The model under review builds one solid part; all positions refer to its coordinate system, in mm. A direction names the side the tool comes from. Give positions to 0.01 mm unless a question says otherwise; leave off trailing zeros. Loops run counter-clockwise (first coordinate to the right, second up) from the corner with the lowest first, then second, coordinate; pieces in that order, holes last. Notation, with made-up numbers: M 1,-11 L 46,-11 A20 ccw 46,22 Z; hole C 9.5,-0.75 d2. An arc over 180 degrees is marked long. Return JSON: item names as keys, results as strings.
```python
from build123d import *

# Parameters (mm, degrees)
F1_DEPTH      = 1200
F2_W          = 30
F2_H          = 30
F3_DEPTH      = 865
F5_W          = 660
F5_H          = 30
F6_DEPTH      = 1085
F6_DEPTH_BACK = 55
F7_W          = 660
F7_H          = 30
F8_DEPTH      = 1085
F8_DEPTH_BACK = 55


with BuildPart() as f1:
    # F0 (on Right) → F1 (new body)
    with BuildSketch(Plane.YZ):
        Polygon((0, 30), (0, 0), (790, 0), (790, 130), (788, 130), (788, 30), align=None)
    extrude(amount=F1_DEPTH)

    # F2 (on face) → F3 (join)
    with BuildSketch(Plane(origin=(0, 0, 0), x_dir=(1, 0, 0), z_dir=(0, 0, -1))):
        with Locations((45, -45)):
            Rectangle(F2_W, F2_H)
        with Locations((1155, -45)):
            Rectangle(F2_W, F2_H)
        with Locations((1155, -675)):
            Rectangle(F2_W, F2_H)
        with Locations((45, -675)):
            Rectangle(F2_W, F2_H)
    extrude(amount=F3_DEPTH)

    # F5 (on offset) → F6 (join, two sides)
    with BuildSketch(Plane.YZ.offset(85)) as f6_sk:
        with Locations((360, -730)):
            Rectangle(F5_W, F5_H)
    extrude(amount=F6_DEPTH)
    extrude(f6_sk.sketch, amount=-F6_DEPTH_BACK)

    # F7 (on offset) → F8 (join, two sides)
    with BuildSketch(Plane.YZ.offset(85)) as f8_sk:
        with Locations((360, -357.5)):
            Rectangle(F7_W, F7_H)
    extrude(amount=F8_DEPTH)
    extrude(f8_sk.sketch, amount=-F8_DEPTH_BACK)


solid = f1.part
```
1) Wall thickness on L1, parallel to Z at x = 1009, y = 583; L2, parallel to Y at x = 1149.5, z = -134; L3, parallel to X at y = 586, z = -730.5: over which ranges is each line inside the solid? List them lowest first. Write a range as from..to.
From the geometry:
{"L1": "-745..-715, -372.5..-342.5, 0..30", "L2": "30..60, 660..690", "L3": "30..1170"}
2) Consider section B-B on z = -537.5. Write out the cut boundary in (x, y).
From the geometry:
{"outline": "M 30,30 L 60,30 L 60,60 L 30,60 Z; M 30,660 L 60,660 L 60,690 L 30,690 Z; M 1140,30 L 1170,30 L 1170,60 L 1140,60 Z; M 1140,660 L 1170,660 L 1170,690 L 1140,690 Z"}
3) Consider section C-C on y = 230. Write out the cut boundary in (x, z), then the cut area to 3 significant figures.
From the geometry:
{"outline": "M 0,0 L 1200,0 L 1200,30 L 0,30 Z; M 30,-745 L 1170,-745 L 1170,-715 L 30,-715 Z; M 30,-372.5 L 1170,-372.5 L 1170,-342.5 L 30,-342.5 Z", "area": "104,000 mm²"}
4) The part is to be moulded in two halves that separate along X. For faces 1 (the face through (1140, 45, -804)), 2 (the face through (1155, 660, -541)), 3 (the face through (1170, 358, -366)), say which applies: released by +X, released by -X, zero draft, split by the parting line, or undercut.
From the geometry:
{"face 1": "undercut", "face 2": "zero draft", "face 3": "released by +X"}
5) Tool access review of faces 4 (the face through (60, 675, -804)), 5 (the face through (1155, 660, -804)), 6 (the face through (30, 358, -366)), 7 (the face through (45, 60, -169)), 8 (the face through (1140, 675, -541)): name each direction out of +Z, -Z, +X, -X, +Y, -Y from which nothing blocks a thin tool from reaching the whole face with its end or side.
From the geometry:
{"face 4": "-Z, +Y, -Y", "face 5": "-Z, +X, -X", "face 6": "-Z, -X, +Y, -Y", "face 7": "+X, -X", "face 8": "+Y, -Y"}
6) Consider section D-D on y = 733.5. Write out the cut boundary in (x, z), then the cut area to 3 significant figures.
From the geometry:
{"outline": "M 0,0 L 1200,0 L 1200,30 L 0,30 Z", "area": "36,000 mm²"}
7) Consider section A-A on x = 808.5. Write out the cut boundary in (y, z).
From the geometry:
{"outline": "M 0,0 L 790,0 L 790,130 L 788,130 L 788,30 L 0,30 Z; M 30,-745 L 690,-745 L 690,-715 L 30,-715 Z; M 30,-372.5 L 690,-372.5 L 690,-342.5 L 30,-342.5 Z"}
8) Insertion check: pin 1 (12 mm diameter, centred on x = 838, z = -375, fed in from -Y); pin 2 (9 mm diameter, centred on x = 43, z = -775.5, fed in from +Y); pin 3 (12 mm diameter, centred on x = 375, y = 590.5, fed in from +Z). Each pin has a flat end and moves straight along its axis. Give the tip position at first contact, or say it passes through.
From the geometry:
{"pin 1": "y = 30", "pin 2": "y = 690", "pin 3": "z = 30"}
